from build123d import *

# Parameters (mm, degrees)
MODEL_R                 = 2.45
SALIENTE_EXTRUIR1_DEPTH = 3


with BuildPart() as part:
    # Model → Saliente-Extruir1 (new body)
    with BuildSketch(Plane.XY):
        with BuildLine():
            Line((47.732278764, 49.864167804), (50.5, 41.75))
            Line((50.5, 41.75), (50.5, 27.75))
            Line((50.5, 27.75), (50.5, 14.75))
            Line((50.5, 14.75), (45.5, 14.75))
            Line((45.5, 14.75), (45.5, 17.75))
            Line((45.5, 17.75), (40.5, 17.75))
            Line((40.5, 17.75), (40.5, 14.75))
            Line((40.5, 14.75), (35.5, 14.75))
            Line((35.5, 14.75), (35.5, 27.75))
            Line((35.5, 27.75), (35.5, 41.75))
            Line((35.5, 41.75), (38.267721236, 49.864167804))
            ThreePointArc((38.267721236, 49.864167804), (43, 53.25), (47.732278764, 49.864167804))
        make_face()
        with Locations((43.348582377, 48.25)):
            Circle(MODEL_R, mode=Mode.SUBTRACT)
    extrude(amount=SALIENTE_EXTRUIR1_DEPTH)


solid = part.part
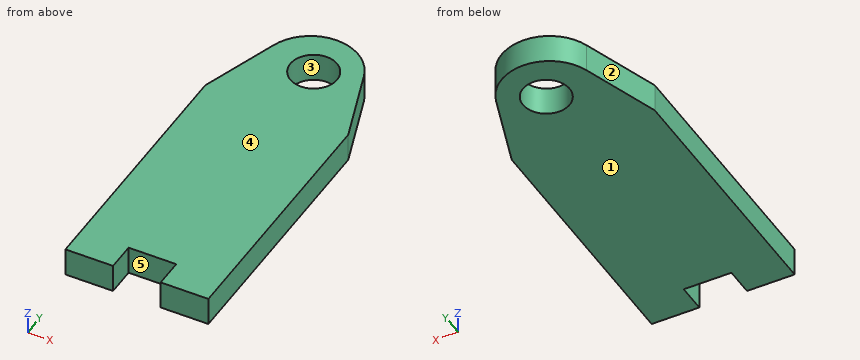
Source: CAD feature listing. Evaluate the final solid. Frame: model axes, mm. Face numbers are marked on the shaded views. A direction names the side the tool comes from. Coordinates: 2 decimals unless noted, no trailing zeros. Loops run counter-clockwise (first coordinate to the right, second up) from the corner with the lowest first, then second, coordinate; pieces in that order, holes last. Notation, with made-up numbers: (10.25, 73.25) -> (57.25, 73.25) arc R6 cw to (57.25, 81.25) -> close; hole circle Ø3 at (-20.75, -32). An arc over 180 degrees is marked (long way). Answer in a Markdown table with one row per item. Add a question column.
Q1. Reachability of the marked faces 4 and 5 from +Z, -Z, +X, -X, +Y, -Y: full face, straight path, thin tool, end or side. Return the list, or none.
Q2. Contact query for flat-ended pins moving along their axis: pin 1 Ø1.5 at (x, z) = (42.5, 1.5) entering from -Y; pin 2 Ø1.5 at (x, z) = (40.5, 0.5) entering from +Y. Output: stop coordinate, or through.
Q3. Ray query, line 1 along Y through (x, z) = (43.25, 2.7); line 2 along Y through (x, z) = (44.5, 0.45); line 3 along X through (y, z) = (48, 2.65). Return the intervals inside material, ascending.
Q4. Section B-B on x = 42.5. Return the cut outline in (y, z), and give its area (3 significant figures).
Q5. Section D-D on x = 39.5. Return the cut outline in (y, z).
Q6. Section A-A on z = 1. Return the cut outline in (x, y), and give its area (3 significant figures).
Q7. Section C-C on y = 48.25. Return the cut outline in (x, z).
Q8. Pull-direction query (X, two-part tool) for the marked faces 1, 2 and 3; classes: pulls with the +X half, pulls with the -X half, needs draft (parallel to the pull), parting line crosses it, or undercut.
Computed values:
| question | item | result |
|---|---|---|
| 1 | face 4 | +Z, +X, -X, +Y, -Y |
| 1 | face 5 | +Z, -Z, -Y |
| 2 | pin 1 | stops at y = 17.75 |
| 2 | pin 2 | stops at y = 52.93 |
| 3 | line 1 | y = 17.75 to 45.8, 50.7 to 53.24 |
| 3 | line 2 | y = 17.75 to 46.09, 50.41 to 53.02 |
| 3 | line 3 | x = 37.63 to 40.91, 45.79 to 48.37 |
| 4 | outline | (17.75, 0) -> (45.95, 0) -> (45.95, 3) -> (17.75, 3) -> close; (50.55, 0) -> (53.22, 0) -> (53.22, 3) -> (50.55, 3) -> close |
| 4 | area | 92.6 mm^2 |
| 5 | outline | (14.75, 0) -> (51.82, 0) -> (51.82, 3) -> (14.75, 3) -> close |
| 6 | outline | (35.5, 14.75) -> (40.5, 14.75) -> (40.5, 17.75) -> (45.5, 17.75) -> (45.5, 14.75) -> (50.5, 14.75) -> (50.5, 41.75) -> (47.73, 49.86) arc R5 ccw to (38.27, 49.86) -> (35.5, 41.75) -> close; hole circle Ø4.9 at (43.35, 48.25) |
| 6 | area | 494 mm^2 |
| 7 | outline | (37.72, 0) -> (40.9, 0) -> (40.9, 3) -> (37.72, 3) -> close; (45.8, 0) -> (48.28, 0) -> (48.28, 3) -> (45.8, 3) -> close |
| 8 | face 1 | needs draft |
| 8 | face 2 | pulls with the -X half |
| 8 | face 3 | undercut |
